```python
from build123d import *

# Parameters (mm, degrees)
SKETCH1_R           = 5.5
SKETCH1_R_2         = 4.5
SKETCH1_R_3         = 4
BOSS_EXTRUDE1_DEPTH = 1
SKETCH1_3_R         = 4.5
SKETCH1_3_R_2       = 4
BOSS_EXTRUDE2_DEPTH = 40
BOSS_EXTRUDE3_START = 39
SKETCH1_4_R         = 5.5
SKETCH1_4_R_2       = 4.5
BOSS_EXTRUDE3_DEPTH = 1
SKETCH2_R           = 1.5
CUT_EXTRUDE1_DEPTH  = 32


with BuildPart() as part:
    # Sketch1 → Boss-Extrude1 (new body)
    with BuildSketch(Plane(origin=(0, 0, 0), x_dir=(1, 0, 0), z_dir=(0, 1, 0))):
        Circle(SKETCH1_R)
        Circle(SKETCH1_R_2, mode=Mode.SUBTRACT)
        Circle(SKETCH1_R_2)
        Circle(SKETCH1_R_3, mode=Mode.SUBTRACT)
    extrude(amount=BOSS_EXTRUDE1_DEPTH)

    # Sketch1_3 → Boss-Extrude2 (add)
    with BuildSketch(Plane(origin=(0, 0, 0), x_dir=(1, 0, 0), z_dir=(0, 1, 0))):
        Circle(SKETCH1_3_R)
        Circle(SKETCH1_3_R_2, mode=Mode.SUBTRACT)
    extrude(amount=BOSS_EXTRUDE2_DEPTH)

    # Sketch1_4 → Boss-Extrude3 (add)
    with BuildSketch(Plane(origin=(0, 0, 0), x_dir=(1, 0, 0), z_dir=(0, 1, 0)).offset(BOSS_EXTRUDE3_START)):
        Circle(SKETCH1_4_R)
        Circle(SKETCH1_4_R_2, mode=Mode.SUBTRACT)
    extrude(amount=BOSS_EXTRUDE3_DEPTH)

    # Sketch2 → Cut-Extrude1 (cut)
    with BuildSketch(Plane(origin=(4.5, 0, 0), x_dir=(0, 0, -1), z_dir=(1, 0, 0))):
        with Locations((0, 10)):
            Circle(SKETCH2_R)
        with Locations((0, 30)):
            Circle(SKETCH2_R)
    extrude(amount=-CUT_EXTRUDE1_DEPTH, mode=Mode.SUBTRACT)


solid = part.part
```
Input: part model. Units: mm. Frame: model coordinates. A direction names the side the tool comes from. Give positions to 0.01 mm unless a question says otherwise; leave off trailing zeros. Loops run counter-clockwise (first coordinate to the right, second up) from the corner with the lowest first, then second, coordinate; pieces in that order, holes last. Notation, with made-up numbers: M -30,-15 L 13,-15 A20 cw 13,17 Z; hole C 30,-8.75 d6. An arc over 180 degrees is marked long. Answer as CSV lines item,"result". Start each with the question number.
1. Section D-D on x = 3. Return loops of the section in (y, z), plus the area to 3 significant figures.
2. Section C-C on y = 20. Return loops of the section in (x, z).
3. Pull-direction query (Z, two-part tool) for faces 1 (the face through (4.11, 31.01, 1.11)), 2 (the face through (-1.19, 39.49, 5.37)), 3 (the face through (-5, 39, 0)); classes: released by +Z, released by -Z, zero draft, split by the parting line, or undercut.
4. Pin query (flat end, axial travel): P1, Ø1.8, axis at y = 30, z = 0, coming from the +X side (1 decimal); P2, Ø4, axis at y = 30, z = 0, coming from the -X side; P3, Ø5, axis at x = -2, y = 22.5, coming from the +Z side; P4, Ø6, axis at x = -1, y = 14.5, coming from the -Z side. Return the tip coordinate at first contact, or that it passes through.
5. Line query: L1, parallel to Y at x = -4.2, z = 0; L2, parallel to Z at x = 0, y = 28.5; L3, parallel to X at y = 38, z = -2. Output: solid intervals per line, ascending.
6. Section B-B on y = 10. Return loops of the section in (x, z), plus the area to 3 significant figures.
7. Section A-A on x = 0. Return loops of the section in (y, z), plus the area to 3 significant figures.
8. Reachability of faces 4 (the face through (-5, 1, 0)), 5 (the face through (3.695, 19.72, 1.532)) from +Z, -Z, +X, -X, +Y, -Y: full face, straight path, thin tool, end or side. Return the list, or none.
Computed values:
1,outline,"M 0,-4.61 L 1,-4.61 L 1,-3.35 L 39,-3.35 L 39,-4.61 L 40,-4.61 L 40,-2.65 L 0,-2.65 Z; M 0,2.65 L 40,2.65 L 40,4.61 L 39,4.61 L 39,3.35 L 1,3.35 L 1,4.61 L 0,4.61 Z"
1,area,"61.7 mm²"
2,outline,"C 0,0 d9; hole C 0,0 d8"
3,face 1,"undercut"
3,face 2,"split by the parting line"
3,face 3,"zero draft"
4,P1,"passes through"
4,P2,"stops at x = -4.5"
4,P3,"stops at z = 4.5"
4,P4,"stops at z = -4.5"
5,L1,"y = 0 to 8.5, 11.5 to 28.5, 31.5 to 40"
5,L2,"z = -4.5 to -4, 4 to 4.5"
5,L3,"x = -4.03 to -3.46, 3.46 to 4.03"
6,outline,"M -4.24,-1.5 A4.5 ccw 4.24,-1.5 L 3.71,-1.5 A4 cw -3.71,-1.5 Z; M -4.24,1.5 L -3.71,1.5 A4 cw 3.71,1.5 L 4.24,1.5 A4.5 ccw Z"
6,area,"10.3 mm²"
7,outline,"M 0,-5.5 L 1,-5.5 L 1,-4.5 L 39,-4.5 L 39,-5.5 L 40,-5.5 L 40,-4 L 0,-4 Z; M 0,4 L 40,4 L 40,5.5 L 39,5.5 L 39,4.5 L 1,4.5 L 1,5.5 L 0,5.5 Z"
7,area,"44.0 mm²"
8,face 4,"none"
8,face 5,"+Y, -Y"
